Here's how the part is built. I have some questions about the finished solid (model axes, mm). A direction names the side the tool comes from. Give positions to 0.01 mm unless a question says otherwise; leave off trailing zeros. Loops run counter-clockwise (first coordinate to the right, second up) from the corner with the lowest first, then second, coordinate; pieces in that order, holes last. Notation, with made-up numbers: (-34, 38.5) - (-13, 38.5) arc R10 ccw to (-13, 52.5) - close; hole circle Ø3 at (-7.5, -23.5). An arc over 180 degrees is marked (long way). Use a Markdown table: item, result.
from build123d import *

# Parameters (mm, degrees)
BOSS_EXTRUDE1_DEPTH = 8
CHAMFER1_SIZE       = 10
CHAMFER1_SIZE2      = 65
CHAMFER2_SIZE       = 65
CHAMFER2_SIZE2      = 10
FILLET2_R           = 15
FILLET3_R           = 50
SKETCH2_R           = 4
CUT_EXTRUDE1_DEPTH  = 80
CUT_EXTRUDE2_DEPTH  = 8


with BuildPart() as part:
    # Sketch1 → Boss-Extrude1 (new body)
    with BuildSketch(Plane.XY):
        Polygon((0, 17.5), (0, 27.5), (-8, 27.5), (-8, 37), (0, 37), (0, 45), (-125, 45), (-125, 22.5), (-125, 0), (0, 0), (0, 8), (-8, 8), (-8, 17.5), align=None)
    extrude(amount=BOSS_EXTRUDE1_DEPTH)

    # Chamfer1
    chamfer1_edges = [part.edges().sort_by_distance(p)[0] for p in [
        (-125, 0, 4),
    ]]
    chamfer1_side = [part.faces().sort_by_distance(p)[0] for p in [
        (-125, 22.5, 4),
    ]]
    chamfer(chamfer1_edges, length=CHAMFER1_SIZE, length2=CHAMFER1_SIZE2, reference=chamfer1_side[0])

    # Chamfer2
    chamfer2_edges = [part.edges().sort_by_distance(p)[0] for p in [
        (-125, 45, 4),
    ]]
    chamfer2_side = [part.faces().sort_by_distance(p)[0] for p in [
        (-62.5, 45, 4),
    ]]
    chamfer(chamfer2_edges, length=CHAMFER2_SIZE, length2=CHAMFER2_SIZE2, reference=chamfer2_side[0])

    # Fillet2
    # the kernel refuses this fillet: 15 mm, written as the material it takes off along each edge
    with BuildSketch(Plane(origin=(-125, 10, -32.171960879), x_dir=(0, 1, 0), z_dir=(0, 0, 1))) as fillet2_piece_1:
        with BuildLine():
            CenterArc((FILLET2_R * 0.857918956767, -FILLET2_R), FILLET2_R, 90, 81.253837737)
            Line((-FILLET2_R * 0.130452740884, -FILLET2_R * 0.847942815746), (0, 0))
            Line((0, 0), (FILLET2_R * 0.857918956767, 0))
        make_face()
    extrude(amount=72.343921757, mode=Mode.SUBTRACT)
    with BuildSketch(Plane(origin=(-125, 35, -32.171960879), x_dir=(0, -1, 0), z_dir=(0, 0, 1))) as fillet2_piece_2:
        with BuildLine():
            CenterArc((FILLET2_R * 0.857918956767, FILLET2_R), FILLET2_R, 188.746162263, 81.253837737)
            Line((-FILLET2_R * 0.130452740884, FILLET2_R * 0.847942815746), (0, 0))
            Line((0, 0), (FILLET2_R * 0.857918956767, 0))
        make_face()
    extrude(amount=72.343921757, mode=Mode.SUBTRACT)

    # Fillet3
    fillet3_edges = [part.edges().sort_by_distance(p)[0] for p in [
        (-60, 0, 4),
        (-60, 45, 4),
    ]]
    fillet(fillet3_edges, radius=FILLET3_R)

    # Sketch2 → Cut-Extrude1 (cut)
    with BuildSketch(Plane.XY.offset(8)):
        with Locations((-110, 22.868784351)):
            Circle(SKETCH2_R)
    extrude(amount=-CUT_EXTRUDE1_DEPTH, mode=Mode.SUBTRACT)

    # Sketch3 → Cut-Extrude2 (cut)
    with BuildSketch(Plane.XY.offset(8)):
        with BuildLine():
            Line((-73, 5.5), (-63, 5.5))
            ThreePointArc((-63, 5.5), (-61.5, 7), (-63, 8.5))
            Line((-63, 8.5), (-73, 8.5))
            ThreePointArc((-73, 8.5), (-74.5, 7), (-73, 5.5))
        make_face()
        with BuildLine():
            Line((-73, 36.5), (-63, 36.5))
            ThreePointArc((-63, 36.5), (-61.5, 38), (-63, 39.5))
            Line((-63, 39.5), (-73, 39.5))
            ThreePointArc((-73, 39.5), (-74.5, 38), (-73, 36.5))
        make_face()
        with BuildLine():
            ThreePointArc((-45, 11.25), (-37.045048712, 14.545048712), (-33.75, 22.5))
            Line((-33.75, 22.5), (-50, 22.5))
            Line((-50, 22.5), (-50, 33.75))
            Line((-50, 33.75), (-55, 33.75))
            ThreePointArc((-55, 33.75), (-66.25, 22.5), (-55, 11.25))
            Line((-55, 11.25), (-45, 11.25))
        make_face()
        with BuildLine():
            Line((-50, 22.5), (-33.75, 22.5))
            ThreePointArc((-33.75, 22.5), (-37.045048712, 30.454951288), (-45, 33.75))
            Line((-45, 33.75), (-50, 33.75))
            Line((-50, 33.75), (-50, 22.5))
        make_face()
        with BuildLine():
            Line((-34.5, 36.5), (-24.5, 36.5))
            ThreePointArc((-24.5, 36.5), (-23, 38), (-24.5, 39.5))
            Line((-24.5, 39.5), (-34.5, 39.5))
            ThreePointArc((-34.5, 39.5), (-36, 38), (-34.5, 36.5))
        make_face()
        with BuildLine():
            Line((-34.5, 5.5), (-24.5, 5.5))
            ThreePointArc((-24.5, 5.5), (-23, 7), (-24.5, 8.5))
            Line((-24.5, 8.5), (-34.5, 8.5))
            ThreePointArc((-34.5, 8.5), (-36, 7), (-34.5, 5.5))
        make_face()
    extrude(amount=-CUT_EXTRUDE2_DEPTH, mode=Mode.SUBTRACT)


solid = part.part
(1) If I drill on line 1 (Y direction, x = -55, z = 3); line 2 (Y direction, x = -66.5, z = 4.5); line 3 (Y direction, x = -42, z = 7.5), over which ranges is the centre line in solid material (lowest first)?
A:
| item | result |
|---|---|
| line 1 | 0 to 11.25, 33.75 to 45 |
| line 2 | 1 to 5.5, 8.5 to 36.5, 39.5 to 44 |
| line 3 | 0 to 11.66, 33.34 to 45 |
(2) Suppose I cut it at D-D on x = -97. Write out the boundary of the cut face in (y, z).
A:
| item | result |
|---|---|
| outline | (5.69, 0) - (39.31, 0) - (39.31, 8) - (5.69, 8) - close |
(3) Will these pins go through, and if not, where does the flat tip stop? pin 1 (4 mm diameter, centred on x = -69, z = 4, fed in from -Y); pin 2 (1 mm diameter, centred on y = 26.5, z = 6.5, fed in from -X); pin 3 (4 mm diameter, centred on x = -112, z = 4, fed in from -Y).
A:
| item | result |
|---|---|
| pin 1 | y = 1.08 |
| pin 2 | x = -124.49 |
| pin 3 | y = 7.69 |
(4) Suppose I cut it at C-C on z = 4.5. Count the separate pieces of the cut face and the enclosed holes in it, plus the area to 3 significant figures.
A:
| item | result |
|---|---|
| separate pieces | 1 |
| enclosed holes | 6 |
| area | 3,930 mm2 |
(5) On a 3-axis mill with a long thin cutter (end or side, diameter ignored), from which of +Z, -Z, +X, -X, +Y, -Y can I reach the whole of each face in a straight line? I mean faces 1 (the face through (-4, 8, 4)), 2 (the face through (-30, 36.5, 4)), 3 (the face through (-88.37, 40.635, 3.944)). Say none if no direction works.
A:
| item | result |
|---|---|
| face 1 | +Z, -Z, +X |
| face 2 | +Z, -Z |
| face 3 | +Z, -Z, -X, +Y |
(6) We'd pull the mould along X, two halves only. Please class faces 4 (the face through (-23, 38, 4)), 5 (the face through (-59.94, 44.86, 4.06)), 6 (the face through (-4, 37, 4)): pulls with the +X half, pulls with the -X half, needs draft (parallel to the pull), parting line crosses it, or undercut.
A:
| item | result |
|---|---|
| face 4 | undercut |
| face 5 | pulls with the -X half |
| face 6 | needs draft |
(7) Suppose I cut it at B-B on x = -39. Write out the boundary of the cut face in (y, z), plus the area to 3 significant figures.
A:
| item | result |
|---|---|
| outline | (0, 0) - (12.98, 0) - (12.98, 8) - (0, 8) - close; (32.02, 0) - (45, 0) - (45, 8) - (32.02, 8) - close |
| area | 208 mm2 |
(8) Suppose I cut it at A-A on y = 20.5. Write out the boundary of the cut face in (x, z).
A:
| item | result |
|---|---|
| outline | (-124.81, 0) - (-113.22, 0) - (-113.22, 8) - (-124.81, 8) - close; (-106.78, 0) - (-66.07, 0) - (-66.07, 8) - (-106.78, 8) - close; (-33.93, 0) - (0, 0) - (0, 8) - (-33.93, 8) - close |
